```python
from build123d import *

# Parameters (mm, degrees)
BOSS_EXTRUDE1_DEPTH = 6.35


with BuildPart() as part:
    # Sketch1 → Boss-Extrude1 (new body)
    with BuildSketch(Plane.XY):
        with BuildLine():
            Line((-73.318041641, -64.069069833), (-83.016400713, -17.165487727))
            ThreePointArc((-83.016400713, -17.165487727), (0, 84.7725), (83.016400713, -17.165487727))
            Line((83.016400713, -17.165487727), (73.318041641, -64.069069833))
            Line((73.318041641, -64.069069833), (64.069069833, -73.318041641))
            Line((64.069069833, -73.318041641), (17.165487727, -83.016400713))
            ThreePointArc((17.165487727, -83.016400713), (0, -84.7725), (-17.165487727, -83.016400713))
            Line((-17.165487727, -83.016400713), (-64.069069833, -73.318041641))
            Line((-64.069069833, -73.318041641), (-73.318041641, -64.069069833))
        make_face()
        with BuildLine():
            Line((63.75441487, -72.734670991), (72.734670991, -63.75441487))
            Line((72.734670991, -63.75441487), (82.394555015, -17.036907295))
            ThreePointArc((82.394555015, -17.036907295), (0, 84.1375), (-82.394555015, -17.036907295))
            Line((-82.394555015, -17.036907295), (-72.734670991, -63.75441487))
            Line((-72.734670991, -63.75441487), (-63.75441487, -72.734670991))
            Line((-63.75441487, -72.734670991), (-17.036907295, -82.394555015))
            ThreePointArc((-17.036907295, -82.394555015), (0, -84.1375), (17.036907295, -82.394555015))
            Line((17.036907295, -82.394555015), (63.75441487, -72.734670991))
        make_face(mode=Mode.SUBTRACT)
    extrude(amount=BOSS_EXTRUDE1_DEPTH)


solid = part.part
```
Geometry check sheet. Reference: the model listing, model coordinates, mm. A direction names the side the tool comes from. Coordinates: 2 decimals unless noted, no trailing zeros. Write each loop counter-clockwise with the first axis right and the second up, starting at its lowest first coordinate (ties: lowest second). Pieces come first, ordered by that corner, then holes. Notation, with made-up numbers: M 62.25,0 L 82.25,0 A23 cw 82.25,25 Z; hole C -31.75,46.25 d1. An arc over 180 degrees is marked long. One line per item, written item: value. Start each with the question number.
(1) Tool access check on faces 1 (the face through (-68.31, -68.18, 3.13)), 2 (the face through (78.235, -40.289, 3.131)). Record the directions out of +Z, -Z, +X, -X, +Y, -Y that give a thin tool (end or side, any length) a straight path to the whole face; none if there is none.
(2) Release check for a two-part mould opening along X. For faces 3 (the face through (40.95, -78.1, 3.13)), 4 (the face through (0.242, -84.772, 3.131)), 5 (the face through (2.09, 84.11, 3.13)), 6 (the face through (-81, -25, 0)) record: released by +X, released by -X, zero draft, split by the parting line, or undercut.
(3) Sectioned sample at A-A, the plane x = 0. Enter the section's corners in (y, z).
(4) Scan lines: line 1 along X through (y, z) = (0, 3); line 2 along X through (y, z) = (59, 0.75); line 3 along Y through (x, z) = (-72, 3.5). Record each from-to range of solid material in increasing order. Write a range as [from, to].
(5) Depth check by flat-ended pin: pin 1 (1 mm diameter, centred on y = -55.5, z = 5, fed in from -X); pin 2 (3 mm diameter, centred on y = -35, z = 3.5, fed in from -X); pin 3 (1.5 mm diameter, centred on x = 44, z = 2, fed in from +Y). Enter the tip coordinate at first touch or a pass-through.
(6) Sectioned sample at C-C, the plane z = 3.5. Enter the section's corners in (x, y) (1 decimal).
Filled sheet:
1. face 1: +Z, -Z
1. face 2: +Z, -Z, +X, -Y
2. face 3: released by +X
2. face 4: split by the parting line
2. face 5: undercut
2. face 6: zero draft
3. outline: M -84.77,0 L -84.14,0 L -84.14,6.35 L -84.77,6.35 Z; M 84.14,0 L 84.77,0 L 84.77,6.35 L 84.14,6.35 Z
4. line 1: [-84.77, -84.14], [84.14, 84.77]
4. line 2: [-60.87, -59.98], [59.98, 60.87]
4. line 3: [-65.39, -64.49], [43.53, 44.75]
5. pin 1: x = -75.19
5. pin 2: x = -79.64
5. pin 3: y = 72.91
6. outline: M -83,-17.2 L -73.3,-64.1 L -64.1,-73.3 L -17.2,-83 A84.8 ccw 17.2,-83 L 64.1,-73.3 L 73.3,-64.1 L 83,-17.2 A84.8 ccw long Z; hole M -82.4,-17 L -72.7,-63.8 L -63.8,-72.7 L -17,-82.4 A84.1 ccw 17,-82.4 L 63.8,-72.7 L 72.7,-63.8 L 82.4,-17 A84.1 ccw long Z
